```python
from build123d import *


with BuildPart() as part:
    # Sketch1 → Revolve1 (revolve)
    with BuildSketch(Plane.XY):
        Polygon((0, 34.572999671), (0, 13.572999671), (5, 13.572999671), (5, 17.52594584), (8.402394853, 23.52594584), (8.402394853, 29.111258282), (6.350943696, 31.572999671), (3.5, 31.572999671), (3.5, 32.572999671), (2.5, 32.572999671), (2.5, 34.572999671), align=None)
    revolve1 = revolve(axis=Axis((0, 34.572999671, 0), (0, -1, 0)))

    # Mirror1: Revolve1 across plane
    add(revolve1.mirror(Plane.ZX.offset(13.572999671)))


solid = part.part
```
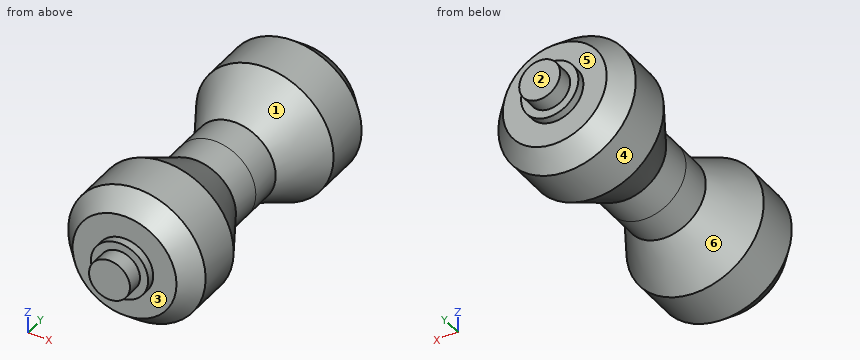
Geometry: final body of the model. Coordinates: model frame, mm. Face numbers are marked on the shaded views. A direction names the side the tool comes from. Give positions to 0.01 mm unless a question says otherwise; leave off trailing zeros. Order: outer loops, then holes, each group sorted by start corner. A loop starts at its lowest first (then second) coordinate and runs counter-clockwise, first axis right, second up. Notation, with made-up numbers: (3.25, -32.5) -> (40.25, -32.5) arc R22 ccw to (40.25, 3.5) -> close; hole circle Ø1 at (84, 33). An arc over 180 degrees is marked (long way). Write each question's results on one line, items separated by ' | '. Start each with the question number.
1) First-contact query: pin 1 (1 mm diameter, centred on x = -4, z = -4, fed in from +Y); pin 2 (4 mm diameter, centred on x = -5.5, z = 4, fed in from -Y); pin 3 (2 mm diameter, centred on x = 3.5, z = 2, fed in from +Y). Flat tips, straight axial feed; report the tip coordinate or a pass-through.
2) Set-up query: the marked faces 1, 2 and 3. Return all of +Z, -Z, +X, -X, +Y, -Y with unobstructed straight access to the full face (end or side cutting, diameter ignored); none if empty.
3) Line query: line 1 (Y direction, x = 1.75, z = 4.5); line 2 (Y direction, x = 7, z = 2.5); line 3 (Y direction, x = 0.5, z = 7). Output: solid intervals per line, ascending. Write a range as from..to.
4) Draft query along Y for the marked faces 4, 5 and 6. Return one class per face: pulls with the +Y half, pulls with the -Y half, needs draft (parallel to the pull), parting line crosses it, or undercut.
5) Section D-D (y = 22.5). Return loops of the section in (x, z).
6) Section C-C (y = -0.5). Return loops of the section in (x, z).
Calculated:
1) pin 1: y = 31.57 | pin 2: y = -4.43 | pin 3: y = 32.57
2) face 1: none | face 2: +Z, -Z, +X, -X, +Y | face 3: -Y
3) line 1: -4.43..31.57 | line 2: -3.13..5.33, 21.82..30.27 | line 3: -3.63..6.06, 21.08..30.77
4) face 4: needs draft | face 5: pulls with the +Y half | face 6: undercut
5) outline: circle Ø15.64 at (0, 0)
6) outline: circle Ø16.8 at (0, 0)
